Model file for the job. Use its own axes, mm. Face numbers are marked on the shaded views. Give positions to 0.01 mm unless a question says otherwise; leave off trailing zeros. Loops run counter-clockwise (first coordinate to the right, second up) from the corner with the lowest first, then second, coordinate; pieces in that order, holes last. Notation, with made-up numbers: (15, 81.5) - (74, 81.5) arc R21 ccw to (74, 111.5) - close; hole circle Ø1 at (14.5, -7.75). An arc over 180 degrees is marked (long way). Use a Markdown table: item, result.
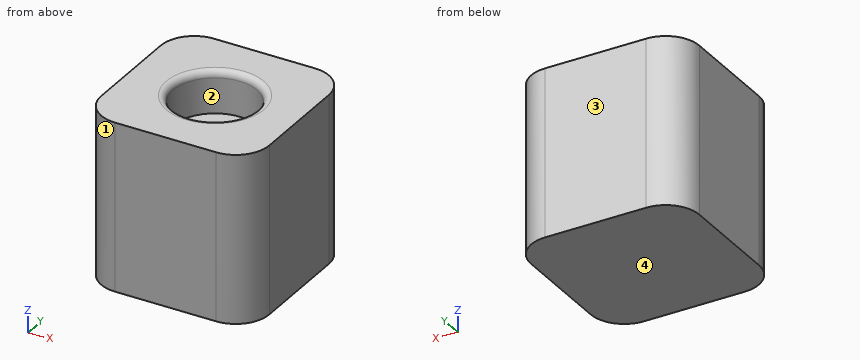
from build123d import *

# Parameters (mm, degrees)
SKETCH_W     = 50
SKETCH_H     = 50
PAD_DEPTH    = 50
SKETCH001_R  = 12.5
POCKET_DEPTH = 12.5
FILLET_R     = 10
FILLET001_R  = 2


with BuildPart() as part:
    # Sketch → Pad (new body)
    with BuildSketch(Plane.XY):
        Rectangle(SKETCH_W, SKETCH_H)
    extrude(amount=PAD_DEPTH)

    # Sketch001 (on Face6 of Pad) → Pocket (cut)
    with BuildSketch(Plane.XY.offset(50)):
        Circle(SKETCH001_R)
    extrude(amount=-POCKET_DEPTH, mode=Mode.SUBTRACT)

    # Fillet
    fillet_edges = [part.edges().sort_by_distance(p)[0] for p in [
        (-25, -25, 25),
        (-25, 25, 25),
        (25, -25, 25),
        (25, 25, 25),
    ]]
    fillet(fillet_edges, radius=FILLET_R)

    # Fillet001
    fillet001_edges = [part.edges().sort_by_distance(p)[0] for p in [
        (-12.5, 0, 50),
    ]]
    fillet(fillet001_edges, radius=FILLET001_R)


solid = part.part
(1) Slice it at C-C, the plane z = 10.5. Write the cut outline in (x, y).
Computed:
| item | result |
|---|---|
| outline | (-25, -15) arc R10 ccw to (-15, -25) - (15, -25) arc R10 ccw to (25, -15) - (25, 15) arc R10 ccw to (15, 25) - (-15, 25) arc R10 ccw to (-25, 15) - close |
(2) Pin check, flat tip, straight feed: P1, Ø12.5, axis at x = 4.5, y = 0, coming from the +Z side. Stop position of the tip, or through.
Computed:
| item | result |
|---|---|
| P1 | z = 37.5 |
(3) Slice it at B-B, the plane y = 0. Write the cut outline in (x, z).
Computed:
| item | result |
|---|---|
| outline | (-25, 0) - (25, 0) - (25, 50) - (14.5, 50) arc R2 ccw to (12.5, 48) - (12.5, 37.5) - (-12.5, 37.5) - (-12.5, 48) arc R2 ccw to (-14.5, 50) - (-25, 50) - close |
(4) Slice it at A-A, the plane z = 45. Write the cut outline in (x, y).
Computed:
| item | result |
|---|---|
| outline | (-25, -15) arc R10 ccw to (-15, -25) - (15, -25) arc R10 ccw to (25, -15) - (25, 15) arc R10 ccw to (15, 25) - (-15, 25) arc R10 ccw to (-25, 15) - close; hole circle Ø25 at (0, 0) |
(5) Drill centre lines: probe 1 along Y at (x, z) = (0, 45); probe 2 along X at (y, z) = (-2, 47); probe 3 along Y at (x, z) = (5, 40). Where is each one in solid material? Low to high. Write a range as [from, to].
Computed:
| item | result |
|---|---|
| probe 1 | [-25, -12.5], [12.5, 25] |
| probe 2 | [-25, -12.34], [12.34, 25] |
| probe 3 | [-25, -11.46], [11.46, 25] |
(6) Mould opens along Y. For the marked faces 1, 2, 3 and 4 say: pulls with the +Y half, pulls with the -Y half, needs draft (parallel to the pull), parting line crosses it, or undercut.
Computed:
| item | result |
|---|---|
| face 1 | pulls with the -Y half |
| face 2 | undercut |
| face 3 | pulls with the +Y half |
| face 4 | needs draft |
